The model under review builds one solid part; all positions refer to its coordinate system, in mm. A direction names the side the tool comes from. Coordinates: 2 decimals unless noted, no trailing zeros. Answer in a Markdown table with one row per item.
Autodesk Inventor part; units mm, degrees
ref_plane "YZ Plane" through (0, 0, 0) normal (1, 0, 0) x (0, 1, 0)
ref_plane "XZ Plane" through (0, 0, 0) normal (0, 1, 0) x (-1, 0, 0)
ref_plane "XY Plane" through (0, 0, 0) normal (0, 0, 1) x (1, 0, 0)
sketch "Sketch20" plane through (0, 0, 0) normal (0, 1, 0) x (-1, 0, 0)
  line L0 (1.5185, -0.8925) -> (-3.5615, -0.8925)
  line L1 (-3.5615, -0.8925) -> (-3.5615, 11.8075)
  line L2 (-3.5615, 11.8075) -> (1.5185, 11.8075)
  line L3 (1.5185, 11.8075) -> (1.5185, -0.8925)
  line L4 (1.5185, 4.9634) -> (-3.5615, 4.9634)
  point P0 (0, 0)
  dimension "d56" = 5.08
  dimension "d57" = 12.7
extrude "Extrusion7" add sketch "Sketch20" along normal blind 2.54 contours L0 L1 L4 L3
extrude "Extrusion8" add sketch "Sketch20" along normal blind 6.35 contours L4 L1 L2 L3
sketch "Sketch21" plane through (0, 2.54, 0) normal (0, 1, 0) x (1, 0, 0)
  line L0 (3.5615, 0.8925) -> (-1.5185, 0.8925)
  line L1 (-1.5185, 0.8925) -> (-1.5185, -4.9634)
  point P0 (0, 0)
  point P1 (1.0215, -1.6475)
  dimension "d62" = 2.54
  dimension "d63" = 2.54
hole "Hole5" at (1.0215, 2.54, 1.6475) direction (0, -1, 0) diameter 3.175 end through all
sketch "Sketch22" plane through (3.5615, 0, -0.8925) normal (1, 0, 0) x (0, 0, -1)
  line L0 (-12.7, 6.35) -> (-5.8558, 6.35)
  line L1 (-12.7, 0) -> (-12.7, 6.35)
  point P0 (-0.8925, 0)
  point P1 (-8.89, 3.175)
  dimension "d71" = 3.175
  dimension "d72" = 3.81
hole "Hole6" at (3.5615, 3.175, 7.9975) direction (-1, 0, 0) diameter 2.85 end through all
sketch "Sketch23" plane through (3.5615, 0, -0.8925) normal (1, 0, 0) x (0, 0, -1)
  line L0 (-5.8558, 2.54) -> (-5.8558, 6.35)
  line L1 (-5.8558, 2.54) -> (-5.8558, 0)
  line L2 (-12.7, 0) -> (0, 0)
  line L3 (-5.8558, 2.54) -> (0, 2.54)
  line L4 (-5.8558, 2.54) -> (0, 2.54)
  line L5 (0, 2.54) -> (0, 0)
  point P0 (-0.8925, 0)
extrude "Extrusion9" add sketch "Sketch23" along normal blind 6.8326
sketch "Sketch24" plane through (0, 2.54, 0) normal (0, 1, 0) x (1, 0, 0)
  line L0 (3.5615, -4.9634) -> (10.3941, -4.9634)
  line L1 (3.5615, -4.9634) -> (3.5615, 0.8925)
  line L2 (-1.5185, 0.8925) -> (10.3941, 0.8925)
  line L3 (3.5615, 0.8925) -> (10.3941, 0.8925)
  line L4 (3.5615, -11.8075) -> (3.5615, -4.9634)
  line L5 (10.3941, -4.9634) -> (3.5615, -4.9634)
  line L6 (3.5615, -4.9634) -> (10.4876, -4.9634)
  line L7 (10.4876, -4.9634) -> (10.3941, -4.9634)
  line L8 (10.3941, -4.9634) -> (10.3941, 0.807)
  line L9 (10.3941, 0.807) -> (10.3941, 0.8925)
  point P0 (0, 0)
extrude "Extrusion10" add sketch "Sketch24" along normal blind 3.81
sketch "Sketch25" plane through (-1.5185, 0, -0.8925) normal (0, 0, -1) x (-1, 0, 0)
  line L0 (-11.9126, 6.35) -> (-5.08, 6.35)
  line L1 (-11.9126, 0) -> (-11.9126, 6.35)
  point P0 (-1.5185, 0)
  point P1 (-8.5968, 3.06)
  dimension "d84" = 3.29
  dimension "d85" = 3.3158
hole "Hole7" at (7.0783, 3.06, -0.8925) direction (0, 0, 1) diameter 2.85 end through all
properties part number "fileholddub"
Item 1: We need section B-B, the plane z = 2.25. State how many separate pieces and enclosed holes the cut face has, then the cut area to 3 significant figures.
Check values:
| item | result |
|---|---|
| separate pieces | 2 |
| enclosed holes | 1 |
| area | 42.4 mm^2 |
Item 2: Mouldability with a two-part tool opening along Y and no side actions: class faces 4 (the face through (8.47, 2.75, 2.08)), 5 (the face through (3.562, 4, 2)), 6 (the face through (3, 0, 4)) as +Y half, -Y half, draft (parallel to the pull), parting line (faces both ways), or undercut.
Check values:
| item | result |
|---|---|
| face 4 | undercut |
| face 5 | draft |
| face 6 | -Y half |
Item 3: To check wall thickness, follow line 1 (X direction, y = 3.06, z = 0.5); line 2 (Y direction, x = 0, z = 4.5); line 3 (X direction, y = 2.75, z = 6.5). State the ranges of each line that lie inside material, in increasing order. Write a range as from..to.
Check values:
| item | result |
|---|---|
| line 1 | 3.56..5.65, 8.5..10.39 |
| line 2 | 0..2.54 |
| line 3 | -1.52..3.56 |
Item 4: Tool access review of faces 1 (the face through (1, 6.35, 8)), 2 (the face through (1, 2.54, 3.4)), 3 (the face through (3.562, 3, 10)): name each direction out of +Z, -Z, +X, -X, +Y, -Y from which nothing blocks a thin tool from reaching the whole face with its end or side.
Check values:
| item | result |
|---|---|
| face 1 | +Z, -Z, +X, -X, +Y |
| face 2 | -Z, -X, +Y |
| face 3 | +Z, +X, +Y, -Y |
Item 5: Clearance check with flat-ended pins moving along their axes: pin 1 Ø1.5 at (x, z) = (2, 2) entering from +Y; pin 2 Ø3 at (x, y) = (6.5, 5) entering from +Z; pin 3 Ø1.1 at (x, y) = (1.5, 3.5) entering from -Z. State where each tip first meets the part, or that it passes through.
Check values:
| item | result |
|---|---|
| pin 1 | y = 2.54 |
| pin 2 | z = 4.96 |
| pin 3 | z = 4.96 |
